Autodesk Inventor part; units mm, degrees
ref_plane "YZ Plane" through (0, 0, 0) normal (1, 0, 0) x (0, 1, 0)
ref_plane "XZ Plane" through (0, 0, 0) normal (0, 1, 0) x (-1, 0, 0)
ref_plane "XY Plane" through (0, 0, 0) normal (0, 0, 1) x (1, 0, 0)
ref_plane "Work Plane1" through (0, 0, 0) normal (0, 0, 1) x (1, 0, 0)
sketch "Sketch1" plane through (0, 0, 0) normal (0, 0, 1) x (1, 0, 0)
  line L0 (230.575, 85.4) -> (230.575, 135.4)
  line L1 (-46.45, 135.4) -> (-46.45, 85.4)
  line L2 (58.575, -49.625) -> (108.575, -49.625)
  line L3 (108.575, 227.4) -> (58.575, 227.4)
  line L4 (-622.225, -47.625) -> (228.575, -47.625)
  line L5 (-44.45, 0) -> (-44.45, 225.4)
  line L6 (180.95, 225.4) -> (-44.45, 225.4)
  line L7 (228.575, -47.625) -> (228.575, 1203.175)
  line L8 (-46.45, 85.4) -> (58.575, 85.4)
  line L9 (108.575, 85.4) -> (230.575, 85.4)
  line L10 (108.575, -49.625) -> (108.575, 85.4)
  line L11 (108.575, 135.4) -> (108.575, 227.4)
  line L12 (58.575, 227.4) -> (58.575, 135.4)
  line L13 (58.575, 85.4) -> (58.575, -49.625)
  line L14 (230.575, 135.4) -> (108.575, 135.4)
  line L15 (58.575, 135.4) -> (-46.45, 135.4)
  point P0 (0, 0)
  point P1 (83.575, 227.4)
  point P2 (83.575, -49.625)
  dimension "d16" = 2
  dimension "d17" = 2
  dimension "d18" = 2
  dimension "d19" = 2
  dimension "d20" = 92
  dimension "d21" = 122
  dimension "d22" = 105.025
  dimension "d23" = 135.025
  dimension "d24" = 50
  dimension "d25" = 50
  dimension "d26" = 50
extrude "Plate1" add sketch "Sketch1" along normal blind 0.5 contours L9 L7 L14 L0 | L9 L10 L4 L13 L8 L5 L15 L12 L6 L11 L14 L7 | L10 L2 L13 L4 | L6 L12 L3 L11 | L8 L1 L15 L5
sketch "Sketch3" plane through (108.575, -49.125, 0.5) normal (0, -1, 0) x (1, 0, 0)
  line L0 (-50, 0) -> (0, 0)
  line L1 (0, 0) -> (0, 25)
  line L2 (0, 25) -> (-50, 25)
  line L3 (-50, 25) -> (-50, 0)
edge flange "Flange2" height 25 angle 90 thickness 0.5 bend radius 0.5 thickness toward (0, -1, 0) relief tear relief width 0.5 relief depth 0.25 corner gap 0.5 corner form 0 edges at (83.575, -49.625, 0.5) (230.575, 110.4, 0.5) (83.575, 227.4, 0.5) (-46.45, 110.4, 0.5) wall of the first edge with corners at (58.575, -49.125, 0.5) (108.575, -49.125, 0.5) (108.575, -49.125, -24.5) (58.575, -49.125, -24.5)
bend "Bend2"
corner "Corner2"
equation "\"d4\" = Thickness"
equation "\"d27\" = BendReliefWidth"
equation "\"d28\" = BendReliefDepth"
equation "\"d29\" = MinimumRemnant"
equation "\"d30\" = TransitionRadius"
equation "\"d33\" = BendRadius"
equation "\"d34\" = CornerReliefSize"
equation "\"d35\" = GapSize"
equation "\"d36\" = JacobiRadiusSize"
equation "\"BendRadius\" = Thickness"
equation "\"BendReliefWidth\" = Thickness"
equation "\"BendReliefDepth\" = 0.5 * Thickness"
equation "\"CornerReliefSize\" = 4 * Thickness"
equation "\"MinimumRemnant\" = 2 * Thickness"
equation "\"TransitionRadius\" = BendRadius"
equation "\"JacobiRadiusSize\" = BendRadius"
equation "\"GapSize\" = Thickness"
properties part number "Brush_holder"
The listing builds one solid part. Answer for the finished solid, in the listing's coordinates (mm). A direction names the side the tool comes from. Coordinates: 2 decimals unless noted, no trailing zeros. Order: outer loops, then holes, each group sorted by start corner. A loop starts at its lowest first (then second) coordinate and runs counter-clockwise, first axis right, second up.
Q1. Which of the six approach directions +Z, -Z, +X, -X, +Y, -Y give full straight-line access (tool end or side, diameter ignored) to faces 1 (the face through (-45.95, 111, -12)), 2 (the face through (84, 226.9, -12)), 3 (the face through (90, 91, 0)), 4 (the face through (-46.45, 111, -13)), 5 (the face through (90, 91, 0.5))?
Q2. Consider line 1 (X direction, y = 100, z = -2.75) (3 decimals); line 2 (Y direction, x = 67, z = -10) (3 decimals); line 3 (Z direction, x = 181.5, y = 99). Determine where each line is inside the solid, lowest interval first.
Q3. A cutting plane is placed at A-A, the plane z = -17. Write down the section's boundary in (x, y) (3 decimals).
Q4. Given P1, Ø4, axis at x = 87.5, y = 147.5, coming from the -Z side, flat-ended and moving along its own axis, determine where the tip first touches the part or whether it passes through.
Q5. A cutting plane is placed at B-B, the plane y = 132. Write down the section's boundary in (x, z) (3 decimals), and give its area (3 significant figures).
Q6. A cutting plane is placed at C-C, the plane x = 160.5. Write down the section's boundary in (y, z), and give its area (3 significant figures).
Q7. For a pull along X with two mould halves and no side action, classify faces 6 (the face through (83, -49.125, -12)), 7 (the face through (230.575, 110, -13)), 8 (the face through (230.075, 110, -12)) as pulls with the +X half, pulls with the -X half, needs draft (parallel to the pull), parting line crosses it, or undercut.
Q8. A cutting plane is placed at D-D, the plane y = 197. Write down the section's boundary in (x, z) (3 decimals), and give its area (3 significant figures).
Answers follow:
1. face 1: -Z, +Y, -Y
1. face 2: -Z, +X, -X
1. face 3: -Z
1. face 4: +Z, -Z, -X, +Y, -Y
1. face 5: +Z, +X, -X, +Y, -Y
2. line 1: x = -46.45 to -45.95, 230.075 to 230.575
2. line 2: y = -49.625 to -49.125, 226.9 to 227.4
2. line 3: z = 0 to 0.5
3. outline: (-46.45, 85.4) - (-45.95, 85.4) - (-45.95, 135.4) - (-46.45, 135.4) - close; (58.575, -49.625) - (108.575, -49.625) - (108.575, -49.125) - (58.575, -49.125) - close; (58.575, 226.9) - (108.575, 226.9) - (108.575, 227.4) - (58.575, 227.4) - close; (230.075, 85.4) - (230.575, 85.4) - (230.575, 135.4) - (230.075, 135.4) - close
4. P1: stops at z = 0
5. outline: (-46.45, -24.5) - (-45.95, -24.5) - (-45.95, -0.5) arc R0.5 cw to (-45.45, 0) - (229.575, 0) arc R0.5 cw to (230.075, -0.5) - (230.075, -24.5) - (230.575, -24.5) - (230.575, -0.5) arc R1 ccw to (229.575, 0.5) - (-45.45, 0.5) arc R1 ccw to (-46.45, -0.5) - close
5. area: 163 mm2
6. outline: (85.4, 0) - (135.4, 0) - (135.4, 0.5) - (85.4, 0.5) - close
6. area: 25.0 mm2
7. face 6: needs draft
7. face 7: pulls with the +X half
7. face 8: undercut
8. outline: (58.575, 0) - (108.575, 0) - (108.575, 0.5) - (58.575, 0.5) - close
8. area: 25.0 mm2
